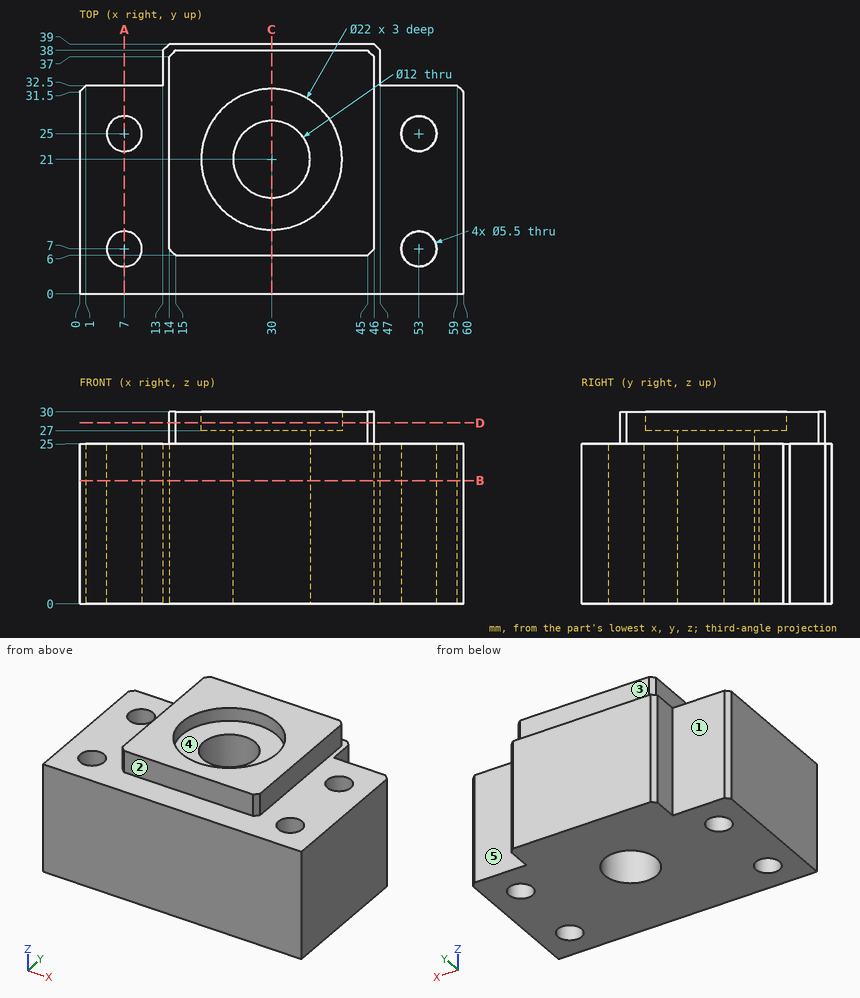
Geometry check sheet. Reference: drawing and pictorial views, mm from the part's lowest x, y, z. A direction names the side the tool comes from. Round coordinates to 2 decimals unless told otherwise and drop trailing zeros. Order: outer loops, then holes, each group sorted by start corner. A loop starts at its lowest first (then second) coordinate and runs counter-clockwise, first axis right, second up. Notation, with made-up numbers: M 39.5,-30 L 98.5,-30 A16 cw 98.5,-22 Z; hole C 9.25,55.25 d7. An arc over 180 degrees is marked long. Answer as CSV lines item,"result".
1) Tool access check on the marked faces 1, 2, 3, 4 and 5. Record the directions out of +Z, -Z, +X, -X, +Y, -Y that give a thin tool (end or side, any length) a straight path to the whole face; none if there is none.
Entries:
face 1,"+Z, -Z, -X, +Y"
face 2,"+Z, +X, -X, -Y"
face 3,"+Z, +X, -X, +Y"
face 4,"+Z"
face 5,"+Z, -Z, +X, +Y"
2) Sectioned sample at B-B on z = 19.25. Record the cut outline in (x, y), and give its area (3 significant figures).
Entries:
outline,"M 0,0 L 60,0 L 60,31.5 L 59,32.5 L 47,32.5 L 47,38 L 46,39 L 14,39 L 13,38 L 13,32.5 L 1,32.5 L 0,31.5 Z; hole C 7,7 d5.5; hole C 7,25 d5.5; hole C 30,21 d12; hole C 53,7 d5.5; hole C 53,25 d5.5"
area,"1,960 mm2"
3) Thickness scan on probe 1 along Y at (x, z) = (53, 10.25); probe 2 along X at (y, z) = (5, 7); probe 3 along Z at (x, y) = (54, 29.5). Record the ranges inside material, lowest first. Write a range as [from, to].
Entries:
probe 1,"[0, 4.25], [9.75, 22.25], [27.75, 32.5]"
probe 2,"[0, 5.11], [8.89, 51.11], [54.89, 60]"
probe 3,"[0, 25]"
4) Gauge pin test, flat ends, axial feed: pin 1 Ø3 at (x, z) = (10.5, 4.5) entering from +Y; pin 2 Ø3 at (y, z) = (36, 11.5) entering from +X; pin 3 Ø2.5 at (x, z) = (30.5, 28.5) entering from -Y. Record the tip position at first contact, or that the pin passes through.
Entries:
pin 1,"y = 32.5"
pin 2,"x = 47"
pin 3,"y = 6"
5) Sectioned sample at C-C on x = 30. Record the cut outline in (y, z), and give its area (3 significant figures).
Entries:
outline,"M 0,0 L 15,0 L 15,27 L 10,27 L 10,30 L 6,30 L 6,25 L 0,25 Z; M 27,0 L 39,0 L 39,25 L 38,25 L 38,30 L 32,30 L 32,27 L 27,27 Z"
area,"745 mm2"
6) Sectioned sample at D-D on z = 28.25. Record the cut outline in (x, y).
Entries:
outline,"M 14,7 L 15,6 L 45,6 L 46,7 L 46,37 L 45,38 L 15,38 L 14,37 Z; hole C 30,21 d22"
7) Sectioned sample at A-A on x = 7. Record the cut outline in (y, z).
Entries:
outline,"M 0,0 L 4.25,0 L 4.25,25 L 0,25 Z; M 9.75,0 L 22.25,0 L 22.25,25 L 9.75,25 Z; M 27.75,0 L 32.5,0 L 32.5,25 L 27.75,25 Z"
